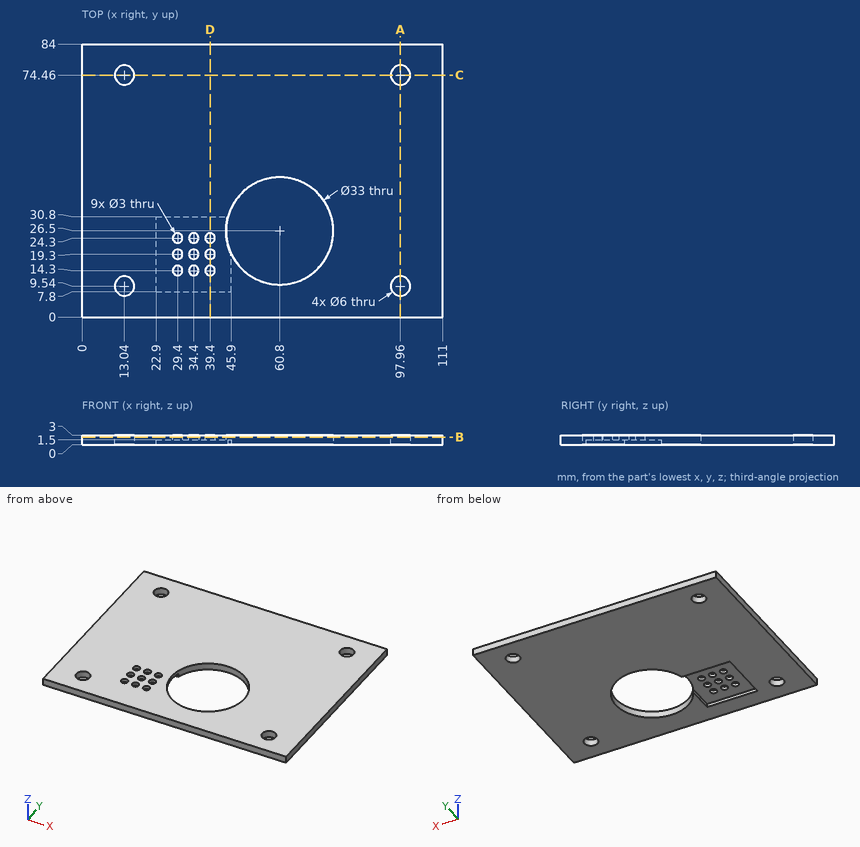
Here's the drawing with two shaded views (mm, measured from the low corner). I have some questions. Give positions to 0.01 mm unless a question says otherwise; leave off trailing zeros. Order: outer loops, then holes, each group sorted by start corner. A loop starts at its lowest first (then second) coordinate and runs counter-clockwise, first axis right, second up. Notation, with made-up numbers: (9, 87.25) -> (36, 87.25) arc R13 cw to (36, 102.25) -> close; hole circle Ø3 at (48, 1.5). An arc over 180 degrees is marked (long way). Use a Markdown table: item, result. Add a question column.
Item 1: Will these pins go through, and if not, where does the flat tip stop? pin 1 (1.6 mm diameter, centred on x = 38.5, z = 1, fed in from -Y); pin 2 (5.5 mm diameter, centred on x = 13.04, y = 9.54, fed in from -Z); pin 3 (3.5 mm diameter, centred on x = 34.4, y = 24.3, fed in from -Z).
Item 2: Imagine slicing it at B-B on z = 2.4. Give the number of separate pieces and of enclosed holes in the cut face, plus the area to 3 significant figures.
Item 3: I need wall thicknesses on line 1 (X direction, y = 9.54, z = 1.6); line 2 (Y direction, x = 39.4, z = 2.05); line 3 (Y direction, x = 99, z = 1.6). Which ranges of each line are inside material? Lowest first, please.
Item 4: Imagine slicing it at C-C on y = 74.46. Please give me the cut outline in (x, z), plus the area to 3 significant figures.
Item 5: Imagine slicing it at A-A on x = 97.96. Please give me the cut outline in (y, z).
Item 6: Imagine slicing it at D-D on x = 39.4. Please give me the cut outline in (y, z), plus the area to 3 significant figures.
Data:
| question | item | result |
|---|---|---|
| 1 | pin 1 | stops at y = 0 |
| 1 | pin 2 | passes through |
| 1 | pin 3 | stops at z = 1.5 |
| 2 | separate pieces | 1 |
| 2 | enclosed holes | 14 |
| 2 | area | 8,290 mm² |
| 3 | line 1 | x = 0 to 10.04, 16.04 to 94.96, 100.96 to 111 |
| 3 | line 2 | y = 0 to 12.8, 15.8 to 17.8, 20.8 to 22.8, 25.8 to 84 |
| 3 | line 3 | y = 0 to 6.73, 12.35 to 71.65, 77.27 to 84 |
| 4 | outline | (0, 0) -> (10.04, 0) -> (10.04, 3) -> (0, 3) -> close; (16.04, 0) -> (94.96, 0) -> (94.96, 3) -> (16.04, 3) -> close; (100.96, 0) -> (111, 0) -> (111, 3) -> (100.96, 3) -> close |
| 4 | area | 297 mm² |
| 5 | outline | (0, 0) -> (6.54, 0) -> (6.54, 3) -> (0, 3) -> close; (12.54, 0) -> (71.46, 0) -> (71.46, 3) -> (12.54, 3) -> close; (77.46, 0) -> (84, 0) -> (84, 3) -> (77.46, 3) -> close |
| 6 | outline | (0, 0) -> (7.8, 0) -> (7.8, 1.5) -> (12.8, 1.5) -> (12.8, 3) -> (0, 3) -> close; (15.8, 1.5) -> (17.8, 1.5) -> (17.8, 3) -> (15.8, 3) -> close; (20.8, 1.5) -> (22.8, 1.5) -> (22.8, 3) -> (20.8, 3) -> close; (25.8, 1.5) -> (30.8, 1.5) -> (30.8, 0) -> (84, 0) -> (84, 3) -> (25.8, 3) -> close |
| 6 | area | 204 mm² |
